from build123d import *

# Parameters (mm, degrees)
SKETCH1_W           = 50.5
SKETCH1_H           = 50.5
SKETCH1_W_2         = 42.5
SKETCH1_H_2         = 42.5
BOSS_EXTRUDE1_DEPTH = 25
SKETCH3_W           = 50.5
SKETCH3_H           = 50.5
SKETCH3_R           = 11.1
SKETCH3_R_2         = 1.6
BOSS_EXTRUDE2_DEPTH = 5
SKETCH6_W           = 30
SKETCH6_H           = 50.5
BOSS_EXTRUDE3_DEPTH = 2
SKETCH7_W           = 30
SKETCH7_H           = 50.5
BOSS_EXTRUDE4_DEPTH = 2
SKETCH5_R           = 1.95
CUT_EXTRUDE1_DEPTH  = 5.7
CUT_EXTRUDE2_DEPTH  = 48.750654446


with BuildPart() as part:
    # Sketch1 → Boss-Extrude1 (new body)
    with BuildSketch(Plane.XY):
        Rectangle(SKETCH1_W, SKETCH1_H)
        Rectangle(SKETCH1_W_2, SKETCH1_H_2, mode=Mode.SUBTRACT)
    extrude(amount=BOSS_EXTRUDE1_DEPTH)

    # Sketch3 → Boss-Extrude2 (add)
    with BuildSketch(Plane.XY.offset(25)):
        Rectangle(SKETCH3_W, SKETCH3_H)
        Circle(SKETCH3_R, mode=Mode.SUBTRACT)
        with Locations((-15.5, 15.5)):
            Circle(SKETCH3_R_2, mode=Mode.SUBTRACT)
        with Locations((15.5, 15.5)):
            Circle(SKETCH3_R_2, mode=Mode.SUBTRACT)
        with Locations((15.5, -15.5)):
            Circle(SKETCH3_R_2, mode=Mode.SUBTRACT)
        with Locations((-15.5, -15.5)):
            Circle(SKETCH3_R_2, mode=Mode.SUBTRACT)
    extrude(amount=BOSS_EXTRUDE2_DEPTH)

    # Sketch6 → Boss-Extrude3 (add)
    with BuildSketch(Plane.ZY.offset(25.25)):
        with Locations((15, 0)):
            Rectangle(SKETCH6_W, SKETCH6_H)
    extrude(amount=BOSS_EXTRUDE3_DEPTH)

    # Sketch7 → Boss-Extrude4 (add)
    with BuildSketch(Plane(origin=(25.25, 0, 0), x_dir=(0, 0, -1), z_dir=(1, 0, 0))):
        with Locations((-15, 0)):
            Rectangle(SKETCH7_W, SKETCH7_H)
    extrude(amount=BOSS_EXTRUDE4_DEPTH)

    # Sketch5 → Cut-Extrude1 (cut)
    with BuildSketch(Plane(origin=(0, -27.3, 0), x_dir=(-1, 0, 0), z_dir=(0, -1, 0))):
        with Locations(Location((-24.25, -3, 0), (0, 0, 180))):
            Circle(SKETCH5_R)
        with Locations(Location((24.25, -3, 0), (0, 0, 270))):
            Circle(SKETCH5_R)
        with Locations(Location((24.25, -27, 0), (0, 0, 180))):
            Circle(SKETCH5_R)
        with Locations(Location((-24.25, -27, 0), (0, 0, 270))):
            Circle(SKETCH5_R)
    extrude(amount=-CUT_EXTRUDE1_DEPTH, mode=Mode.SUBTRACT)

    # Sketch8 → Cut-Extrude2 (cut, through all)
    with BuildSketch(Plane(origin=(0, 0, 0), x_dir=(-1, 0, 0), z_dir=(0, 0, -1))):
        with BuildLine():
            Line((27.25, 25.25), (23.25, 25.25))
            ThreePointArc((23.25, 25.25), (26.078427125, 24.078427125), (27.25, 21.25))
            Line((27.25, 21.25), (27.25, 25.25))
        make_face()
        with BuildLine():
            ThreePointArc((-27.25, 21.25), (-26.078427125, 24.078427125), (-23.25, 25.25))
            Line((-23.25, 25.25), (-27.25, 25.25))
            Line((-27.25, 25.25), (-27.25, 21.25))
        make_face()
    extrude(amount=-CUT_EXTRUDE2_DEPTH, mode=Mode.SUBTRACT)


solid = part.part
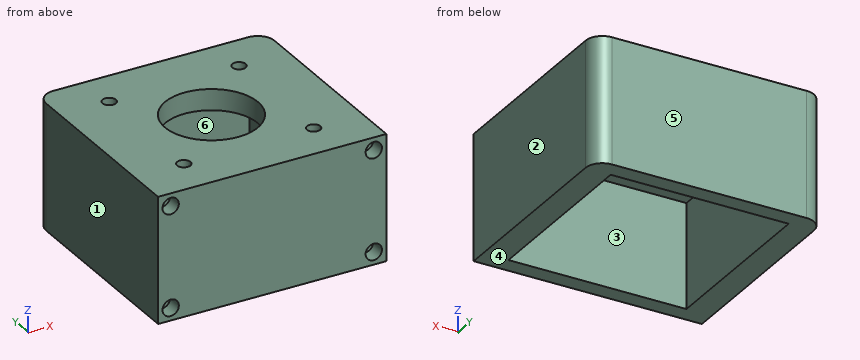
The listing builds one solid part. Answer for the finished solid, in the listing's coordinates (mm). Face numbers are marked on the shaded views. A direction names the side the tool comes from. Round coordinates to 2 decimals unless told otherwise and drop trailing zeros. Order: outer loops, then holes, each group sorted by start corner. A loop starts at its lowest first (then second) coordinate and runs counter-clockwise, first axis right, second up. Notation, with made-up numbers: (46.25, 54) -> (70.25, 54) arc R26 cw to (70.25, 88) -> close; hole circle Ø1 at (62, -29.5). An arc over 180 degrees is marked (long way). Put each result on its own line as item: value.
Q1. Section B-B, the plane z = 27 is taken. Write down the section's boundary in (x, y).
Results list:
outline: (-27.25, -25.25) -> (-26.2, -25.25) -> (-26.2, -21.6) -> (-22.3, -21.6) -> (-22.3, -25.25) -> (22.3, -25.25) -> (22.3, -21.6) -> (26.2, -21.6) -> (26.2, -25.25) -> (27.25, -25.25) -> (27.25, 21.25) arc R4 ccw to (23.25, 25.25) -> (-23.25, 25.25) arc R4 ccw to (-27.25, 21.25) -> close; hole circle Ø3.2 at (-15.5, -15.5); hole circle Ø3.2 at (-15.5, 15.5); hole circle Ø22.2 at (0, 0); hole circle Ø3.2 at (15.5, -15.5); hole circle Ø3.2 at (15.5, 15.5)
Q2. Which of the six approach directions +Z, -Z, +X, -X, +Y, -Y give full straight-line access (tool end or side, diameter ignored) to the marked faces 5 and 6?
Results list:
face 5: +Z, -Z, +X, -X, +Y
face 6: -Z
Q3. Determine the mould class of the marked faces 1, 2, 3 and 4 for opening direction X: pulls with the +X half, pulls with the -X half, needs draft (parallel to the pull), parting line crosses it, or undercut.
Results list:
face 1: pulls with the -X half
face 2: pulls with the +X half
face 3: undercut
face 4: needs draft
Q4. Section A-A, the plane x = -15.5 is taken. Write down the section's boundary in (y, z), and give its area (4 significant figures).
Results list:
outline: (-25.25, 0) -> (-21.25, 0) -> (-21.25, 25) -> (-17.1, 25) -> (-17.1, 30) -> (-25.25, 30) -> close; (-13.9, 25) -> (13.9, 25) -> (13.9, 30) -> (-13.9, 30) -> close; (17.1, 25) -> (21.25, 25) -> (21.25, 0) -> (25.25, 0) -> (25.25, 30) -> (17.1, 30) -> close
area: 420.5 mm^2
Q5. Section C-C, the plane y = 0 is taken. Write down the section's boundary in (x, z).
Results list:
outline: (-27.25, 0) -> (-21.25, 0) -> (-21.25, 25) -> (-11.1, 25) -> (-11.1, 30) -> (-27.25, 30) -> close; (11.1, 25) -> (21.25, 25) -> (21.25, 0) -> (27.25, 0) -> (27.25, 30) -> (11.1, 30) -> close
Q6. Consider line 1 along Y through (x, z) = (15.5, 27.9); line 2 along X through (y, z) = (4, 23.25); line 3 along Y through (x, z) = (18.5, 22.5). Determine where each line is inside the solid, lowest interval first.
Results list:
line 1: -25.25 to -17.1, -13.9 to 13.9, 17.1 to 25.25
line 2: -27.25 to -21.25, 21.25 to 27.25
line 3: -25.25 to -21.25, 21.25 to 25.25
Q7. Each of these flat-tipped pins is pushed along its axis until it touches: P1, Ø1.2, axis at x = 24.5, z = 27.5, coming from the -Y side; P2, Ø8, axis at x = -15.5, y = -2.5, coming from the -Z side. Where does it stop, or does it pass through?
Results list:
P1: y = -21.6
P2: z = 25
Q8. Section D-D, the plane z = 3 is taken. Write down the section's boundary in (x, y), and give its area (3 significant figures).
Results list:
outline: (-27.25, -25.25) -> (-26.2, -25.25) -> (-26.2, -21.6) -> (-22.3, -21.6) -> (-22.3, -25.25) -> (22.3, -25.25) -> (22.3, -21.6) -> (26.2, -21.6) -> (26.2, -25.25) -> (27.25, -25.25) -> (27.25, 21.25) arc R4 ccw to (23.25, 25.25) -> (-23.25, 25.25) arc R4 ccw to (-27.25, 21.25) -> close; hole (-21.25, -21.25) -> (21.25, -21.25) -> (21.25, 21.25) -> (-21.25, 21.25) -> close
area: 911 mm^2
